Geometry check sheet. Reference: the model listing, model coordinates, mm. A direction names the side the tool comes from. Round coordinates to 2 decimals unless told otherwise and drop trailing zeros. Write each loop counter-clockwise with the first axis right and the second up, starting at its lowest first coordinate (ties: lowest second). Pieces come first, ordered by that corner, then holes. Notation, with made-up numbers: (-36.75, 53) -> (-30.75, 53) arc R23 ccw to (-30.75, 78) -> close; hole circle Ø7 at (-8, 75.25). An arc over 180 degrees is marked (long way). Use a Markdown table: item, result.
```python
from build123d import *

# Parameters (mm, degrees)
SKETCH_1_R          = 23.5
EXTRUDE_1_DEPTH     = 4
SKETCH_2_R          = 22.225
EXTRUDE_2_DEPTH     = 3.175
SKETCH_3_R          = 1.6
CUT_EXTRUDE_1_DEPTH = 34.999715072
SKETCH_4_W          = 5
SKETCH_4_H          = 18
CUT_EXTRUDE_2_DEPTH = 34.999715072
SKETCH_5_R          = 1.6
CUT_EXTRUDE_3_DEPTH = 34.999715072


with BuildPart() as part:
    # ｽｹｯﾁ1 → ﾎﾞｽ - 押し出し1 (new body)
    with BuildSketch(Plane.XY):
        Circle(SKETCH_1_R)
    extrude(amount=EXTRUDE_1_DEPTH)

    # ｽｹｯﾁ2 → ﾎﾞｽ - 押し出し2 (add)
    with BuildSketch(Plane(origin=(0, 0, 0), x_dir=(-1, 0, 0), z_dir=(0, 0, -1))):
        Circle(SKETCH_2_R)
    extrude(amount=EXTRUDE_2_DEPTH)

    # ｽｹｯﾁ3 → ｶｯﾄ - 押し出し1 (cut, through all)
    with BuildSketch(Plane(origin=(0, 0, -3.175), x_dir=(-1, 0, 0), z_dir=(0, 0, -1))):
        with Locations((0, 20)):
            Circle(SKETCH_3_R)
        with Locations((20, 0)):
            Circle(SKETCH_3_R)
        with Locations((0, -20)):
            Circle(SKETCH_3_R)
        with Locations((-20, 0)):
            Circle(SKETCH_3_R)
    extrude(amount=-CUT_EXTRUDE_1_DEPTH, mode=Mode.SUBTRACT)

    # ｽｹｯﾁ4 → ｶｯﾄ - 押し出し2 (cut, through all)
    with BuildSketch(Plane(origin=(0, 0, -3.175), x_dir=(-1, 0, 0), z_dir=(0, 0, -1))):
        with Locations((12, 0)):
            Rectangle(SKETCH_4_W, SKETCH_4_H)
        with Locations((-12, 0)):
            Rectangle(SKETCH_4_W, SKETCH_4_H)
    extrude(amount=-CUT_EXTRUDE_2_DEPTH, mode=Mode.SUBTRACT)

    # ｽｹｯﾁ5 → ｶｯﾄ - 押し出し3 (cut, through all)
    with BuildSketch(Plane(origin=(0, 0, -3.175), x_dir=(-1, 0, 0), z_dir=(0, 0, -1))):
        with Locations((-12, 13)):
            Circle(SKETCH_5_R)
        with Locations(Location((-12, -13, 0), (0, 0, 180))):
            Circle(SKETCH_5_R)
        with Locations((12, -13)):
            Circle(SKETCH_5_R)
        with Locations(Location((12, 13, 0), (0, 0, 180))):
            Circle(SKETCH_5_R)
    extrude(amount=-CUT_EXTRUDE_3_DEPTH, mode=Mode.SUBTRACT)


solid = part.part
```
(1) Section check D-D on x = -20. Record the cut outline in (y, z) (3 decimals).
A:
| item | result |
|---|---|
| outline | (-12.339, 0) -> (-9.693, 0) -> (-9.693, -3.175) -> (-1.6, -3.175) -> (-1.6, 4) -> (-12.339, 4) -> close; (1.6, -3.175) -> (9.693, -3.175) -> (9.693, 0) -> (12.339, 0) -> (12.339, 4) -> (1.6, 4) -> close |
(2) Section check A-A on z = -2. State how many separate pieces and enclosed holes the cut face has, plus the area to 3 significant figures.
A:
| item | result |
|---|---|
| separate pieces | 1 |
| enclosed holes | 10 |
| area | 1,310 mm2 |
(3) Thickness scan on line 1 (Y direction, x = 12, z = 0.5); line 2 (Y direction, x = 0, z = 2.75); line 3 (X direction, y = -8, z = -0.5). Record the ranges inside material, lowest first.
A:
| item | result |
|---|---|
| line 1 | y = -20.21 to -14.6, -11.4 to -9, 9 to 11.4, 14.6 to 20.21 |
| line 2 | y = -23.5 to -21.6, -18.4 to 18.4, 21.6 to 23.5 |
| line 3 | x = -20.74 to -14.5, -9.5 to 9.5, 14.5 to 20.74 |
(4) Access from +Z, -Z, +X, -X, +Y, -Y to the whole of each face (thin tool, end or side, straight path). Record for faces 1 (the face through (0, 0, 4)), 2 (the face through (-12, 9, 0)).
A:
| item | result |
|---|---|
| face 1 | +Z, +X, -X, +Y, -Y |
| face 2 | +Z, -Z |
(5) Section check B-B on x = 0. Record the cut outline in (y, z) (3 decimals).
A:
| item | result |
|---|---|
| outline | (-23.5, 0) -> (-22.225, 0) -> (-22.225, -3.175) -> (-21.6, -3.175) -> (-21.6, 4) -> (-23.5, 4) -> close; (-18.4, -3.175) -> (18.4, -3.175) -> (18.4, 4) -> (-18.4, 4) -> close; (21.6, -3.175) -> (22.225, -3.175) -> (22.225, 0) -> (23.5, 0) -> (23.5, 4) -> (21.6, 4) -> close |
(6) Section check C-C on y = 0. Record the cut outline in (x, z) (3 decimals).
A:
| item | result |
|---|---|
| outline | (-23.5, 0) -> (-22.225, 0) -> (-22.225, -3.175) -> (-21.6, -3.175) -> (-21.6, 4) -> (-23.5, 4) -> close; (-18.4, -3.175) -> (-14.5, -3.175) -> (-14.5, 4) -> (-18.4, 4) -> close; (-9.5, -3.175) -> (9.5, -3.175) -> (9.5, 4) -> (-9.5, 4) -> close; (14.5, -3.175) -> (18.4, -3.175) -> (18.4, 4) -> (14.5, 4) -> close; (21.6, -3.175) -> (22.225, -3.175) -> (22.225, 0) -> (23.5, 0) -> (23.5, 4) -> (21.6, 4) -> close |
(7) Gauge pin test, flat ends, axial feed: pin 1 Ø2.5 at (x, z) = (13, 1) entering from -Y; pin 2 Ø1 at (x, z) = (-18.5, 2) entering from +Y; pin 3 Ø3.5 at (y, z) = (-4.5, 0.5) entering from +X. Record the tip position at first contact, or that the pin passes through.
A:
| item | result |
|---|---|
| pin 1 | stops at y = -20.35 |
| pin 2 | stops at y = 15.11 |
| pin 3 | stops at x = 23.34 |
(8) Release check for a two-part mould opening along Y. For faces 3 (the face through (9, -21, 0)), 4 (the face through (22.4, 7.1, 2)), 5 (the face through (-9.5, 0, 0)) record: +Y half, -Y half, draft (parallel to the pull), parting line (faces both ways), or undercut.
A:
| item | result |
|---|---|
| face 3 | draft |
| face 4 | parting line |
| face 5 | undercut |
